Source: three-view drawing plus pictorial views. Frame: mm from the lowest corner of the part. A direction names the side the tool comes from. Round coordinates to 2 decimals unless told otherwise and drop trailing zeros. Loops run counter-clockwise (first coordinate to the right, second up) from the corner with the lowest first, then second, coordinate; pieces in that order, holes last. Notation, with made-up numbers: (-7.5, 51.25) -> (24.5, 51.25) arc R33 ccw to (24.5, 79.25) -> close; hole circle Ø9 at (-31.5, 26). An arc over 180 degrees is marked (long way). Answer as a JSON object with one key per item and string values. Group by question number.
Item 1: Section query D-D on y = 8.75. Return loops of the section in (x, z) (1 decimal).
Item 2: Material intervals for line 1 (Y direction, x = 1.9, z = 2.2) (1 decimal); line 2 (Y direction, x = 0.85, z = 3.25) (1 decimal); line 3 (Z direction, x = 2.65, y = 1), sorted ascending. Write a range as [from, to].
Item 3: Pin query (flat end, axial travel): pin 1 (1.5 mm diameter, centred on y = 3, z = 4, fed in from +X); pin 2 (3 mm diameter, centred on y = 5.5, z = 4.5, fed in from +X); pin 3 (3 mm diameter, centred on x = 4, y = 5.5, fed in from -Z). Return the tip coordinate at first contact, or that it passes through.
Item 4: Section query A-A on y = 1.75. Return loops of the section in (x, z) (1 decimal).
Item 5: Section query C-C on x = 3.95. Return loops of the section in (y, z) (1 decimal).
Item 6: Draft query along Z for the marked faces 1, 2 and 3. Return one class per face: released by +Z, released by -Z, zero draft, split by the parting line, or undercut.
Item 7: Section query B-B on z = 3.1. Return loops of the section in (x, y) (1 decimal).
Item 8: Set-up query: the marked faces 4, 5 and 6. Return all of +Z, -Z, +X, -X, +Y, -Y with unobstructed straight access to the full face (end or side cutting, diameter ignored); none if empty.
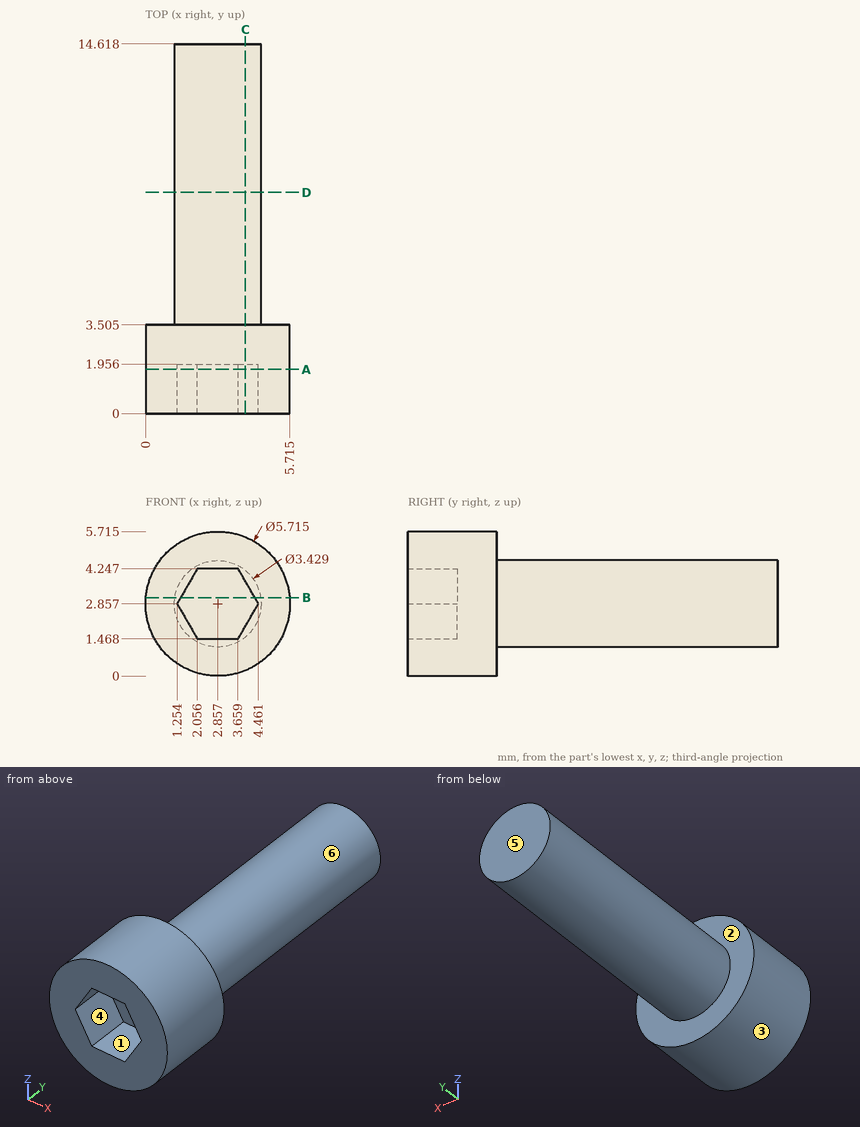
Solved:
{
 "1": {"outline": "circle Ø3.4 at (2.9, 2.9)"},
 "2": {"line 1": "[2, 14.6]", "line 2": "[0, 3.5]", "line 3": "[0.01, 1.47], [4.25, 5.71]"},
 "3": {"pin 1": "x = 5.69", "pin 2": "x = 4.57", "pin 3": "z = 1.14"},
 "4": {"outline": "circle Ø5.7 at (2.9, 2.9); hole (1.3, 2.9) -> (2.1, 1.5) -> (3.7, 1.5) -> (4.5, 2.9) -> (3.7, 4.2) -> (2.1, 4.2) -> close"},
 "5": {"outline": "(0, 0.2) -> (3.5, 0.2) -> (3.5, 1.5) -> (14.6, 1.5) -> (14.6, 4.2) -> (3.5, 4.2) -> (3.5, 5.5) -> (0, 5.5) -> (0, 3.7) -> (2, 3.7) -> (2, 2) -> (0, 2) -> close"},
 "6": {"face 1": "undercut", "face 2": "zero draft", "face 3": "split by the parting line"},
 "7": {"outline": "(0, 0) -> (1.4, 0) -> (1.4, 2) -> (4.3, 2) -> (4.3, 0) -> (5.7, 0) -> (5.7, 3.5) -> (4.6, 3.5) -> (4.6, 14.6) -> (1.2, 14.6) -> (1.2, 3.5) -> (0, 3.5) -> close"},
 "8": {"face 4": "-Y", "face 5": "+Z, -Z, +X, -X, +Y", "face 6": "+Y"}
}
